The model under review builds one solid part; all positions refer to its coordinate system, in mm. Give positions to 0.01 mm unless a question says otherwise; leave off trailing zeros. Loops run counter-clockwise (first coordinate to the right, second up) from the corner with the lowest first, then second, coordinate; pieces in that order, holes last. Notation, with made-up numbers: (24.5, 54.25) - (37.5, 54.25) arc R18 cw to (37.5, 88.25) - close; hole circle Ø1 at (57.5, 89). An arc over 180 degrees is marked (long way). Return JSON: item names as keys, results as strings. Group by question number.
```python
from build123d import *

# Parameters (mm, degrees)
SKETCH5_W                       = 25.4
SKETCH5_H                       = 25.4
BASE_FLANGE1_DEPTH              = 0.7366
EDGE_FLANGE1_START              = 787.4
EDGE_FLANGE1_DEPTH              = 25.4
EDGE_FLANGE1_2_DEPTH            = 25.4
F_5_0MM_DOWEL_HOLE1_D           = 5
F_5_0MM_DOWEL_HOLE1_DEPTH       = 25.4
F_5_0MM_DOWEL_HOLE1_CSINK_D     = 5.05
F_5_0MM_DOWEL_HOLE1_CSINK_ANGLE = 90
F_5_0MM_DOWEL_HOLE1_TIP         = 1.502151548


# Read off the part's stored shape, not the designer's step: Edge-Flange1
# Sheet-metal steps are written as plain solids
with BuildPart() as part:
    # Sketch5 → Base-Flange1 (new body)
    with BuildSketch(Plane(origin=(0, 0, 0), x_dir=(1, 0, 0), z_dir=(0, 1, 0))):
        with Locations((800.1, 101.6)):
            Rectangle(SKETCH5_W, SKETCH5_H)
    extrude(amount=-BASE_FLANGE1_DEPTH)

    # Edge-Flange1 outline → Edge-Flange1 (cut)
    with BuildSketch(Plane.YZ.offset(EDGE_FLANGE1_START)):
        with BuildLine():
            Line((0, -114.3), (-0.391936674, -113.832908061))
            ThreePointArc((-0.391936674, -113.832908061), (-0.647755169, -113.38981743), (-0.7366, -112.885953355))
            Line((-0.7366, -112.885953355), (-0.7366, -114.3))
            Line((-0.7366, -114.3), (0, -114.3))
        make_face()
    edge_flange1 = extrude(amount=EDGE_FLANGE1_DEPTH, mode=Mode.SUBTRACT)

    # Edge-Flange1 2 outline → Edge-Flange1 2 (add)
    with BuildSketch(Plane.YZ.offset(EDGE_FLANGE1_START)):
        with BuildLine():
            Line((0, -112.885953355), (0, -114.3))
            Line((0, -114.3), (113.551037002, -249.62485629))
            Line((113.551037002, -249.62485629), (114.115305339, -249.151378937))
            Line((114.115305339, -249.151378937), (0.172331663, -113.359430708))
            ThreePointArc((0.172331663, -113.359430708), (0.044422416, -113.137885392), (0, -112.885953355))
        make_face()
    edge_flange1_2 = extrude(amount=EDGE_FLANGE1_2_DEPTH)

    # Mirror1: Edge-Flange1, Edge-Flange1 2 across plane
    add(edge_flange1.mirror(Plane.XY.offset(-101.6)), mode=Mode.SUBTRACT)
    add(edge_flange1_2.mirror(Plane.XY.offset(-101.6)))

    # Ø5.0mm Dowel Hole1
    with Locations(Plane(origin=(0, 0, 0), x_dir=(1, 0, 0), z_dir=(0, 1, 0))):
        with Locations((800.1, 107.95), (800.1, 95.25)):
            CounterSinkHole(F_5_0MM_DOWEL_HOLE1_D / 2, F_5_0MM_DOWEL_HOLE1_CSINK_D / 2, depth=F_5_0MM_DOWEL_HOLE1_DEPTH, counter_sink_angle=F_5_0MM_DOWEL_HOLE1_CSINK_ANGLE)
            with Locations((0, 0, -(F_5_0MM_DOWEL_HOLE1_DEPTH + F_5_0MM_DOWEL_HOLE1_TIP / 2))):  # 118° drill point
                Cone(0, F_5_0MM_DOWEL_HOLE1_D / 2, F_5_0MM_DOWEL_HOLE1_TIP, mode=Mode.SUBTRACT)


solid = part.part
```
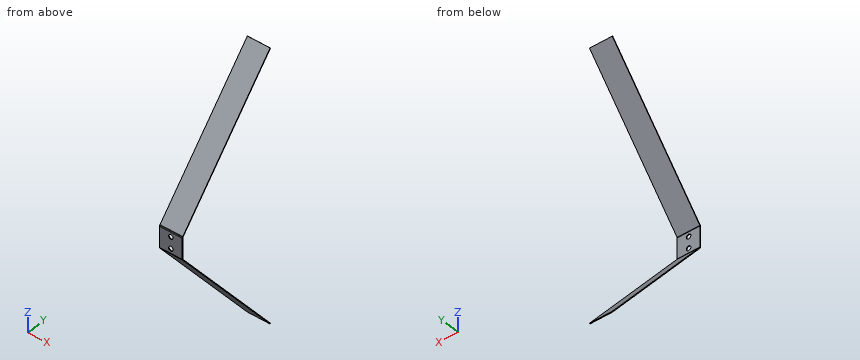
1) For pin 1 Ø2 at (x, y) = (798.5, 68.5) entering from +Z; pin 2 Ø3 at (x, y) = (790.5, 100) entering from +Z; pin 3 Ø2 at (x, y) = (807.5, 47.5) entering from +Z, all flat-tipped, find the tip position at first contact; note any pin that passes through.
2) We need section B-B, the plane y = 90.5. Write out the cut boundary in (x, z), plus the area to 3 significant figures.
3) We need section A-A, the plane x = 807.75. Write out the cut boundary in (y, z).
4) We need section C-C, the plane z = -39. Write out the cut boundary in (x, y).
5) To check wall thickness, follow line 1 (Z direction, x = 800.1, y = -0.35); line 2 (Z direction, x = 800.1, y = -0.45); line 3 (X direction, y = -0.2, z = -95.25). State the ranges of each line that lie inside material, in increasing order.
Findings:
{
 "1": {"pin 1": "stops at z = -6.07", "pin 2": "stops at z = 32.06", "pin 3": "stops at z = -31.1"},
 "2": {"outline": "(787.4, -222.15) - (812.8, -222.15) - (812.8, -221.01) - (787.4, -221.01) - close; (787.4, 17.81) - (812.8, 17.81) - (812.8, 18.95) - (787.4, 18.95) - close", "area": "58.2 mm^2"},
 "3": {"outline": "(-0.74, -112.89) arc R1.47 ccw to (-0.39, -113.83) - (113.55, -249.62) - (114.12, -249.15) - (0.17, -113.36) arc R0.74 cw to (0, -112.89) - (0, -90.31) arc R0.74 cw to (0.17, -89.84) - (114.12, 45.95) - (113.55, 46.42) - (-0.39, -89.37) arc R1.47 ccw to (-0.74, -90.31) - close"},
 "4": {"outline": "(787.4, 41.87) - (812.8, 41.87) - (812.8, 42.83) - (787.4, 42.83) - close"},
 "5": {"line 1": "z = -113.88 to -110.45, -105.45 to -97.75, -92.75 to -89.32", "line 2": "z = -113.76 to -110.45, -105.45 to -97.75, -92.75 to -89.44", "line 3": "x = 787.4 to 797.6, 802.6 to 812.8"}
}
